Could you check a few things on this model? Use its own coordinates, in mm. Give positions to 0.01 mm unless a question says otherwise; leave off trailing zeros. Write each loop counter-clockwise with the first axis right and the second up, starting at its lowest first coordinate (ties: lowest second). Pieces come first, ordered by that corner, then holes. Notation, with made-up numbers: (58.5, 26.5) -> (90.5, 26.5) arc R12 cw to (90.5, 47.5) -> close; hole circle Ø5 at (-27.5, -22). An arc over 180 degrees is marked (long way). One line per question, with ' | ' between items.
from build123d import *

# Parameters (mm, degrees)
ESQUISSE1_W             = 370
ESQUISSE1_H             = 180
BOSS_EXTRU_1_DEPTH      = 6
ESQUISSE2_W             = 6
ESQUISSE2_H             = 30
ENL_V_MAT_EXTRU_1_DEPTH = 10
CONG_1_R                = 10


with BuildPart() as part:
    # Esquisse1 → Boss.-Extru.1 (new body)
    with BuildSketch(Plane.XY):
        with Locations((185, 90)):
            Rectangle(ESQUISSE1_W, ESQUISSE1_H)
    extrude(amount=BOSS_EXTRU_1_DEPTH)

    # Esquisse2 → Enlèv. mat.-Extru.1 (cut)
    with BuildSketch(Plane.XY.offset(6)):
        with Locations((8, 55)):
            Rectangle(ESQUISSE2_W, ESQUISSE2_H)
        with Locations((8, 125)):
            Rectangle(ESQUISSE2_W, ESQUISSE2_H)
        with Locations((362, 125)):
            Rectangle(ESQUISSE2_W, ESQUISSE2_H)
        with Locations((362, 55)):
            Rectangle(ESQUISSE2_W, ESQUISSE2_H)
    extrude(amount=-ENL_V_MAT_EXTRU_1_DEPTH, mode=Mode.SUBTRACT)

    # Congé1
    cong_1_edges = [part.edges().sort_by_distance(p)[0] for p in [
        (0, 180, 3),
        (370, 180, 3),
        (370, 0, 3),
        (0, 0, 3),
    ]]
    fillet(cong_1_edges, radius=CONG_1_R)


solid = part.part
Q1. Will these pins go through, and if not, where does the flat tip stop? pin 1 (1.8 mm diameter, centred on x = 363.5, z = 4, fed in from +Y); pin 2 (3 mm diameter, centred on x = 363, z = 1.5, fed in from -Y); pin 3 (1.8 mm diameter, centred on x = 7, z = 1.5, fed in from -Y).
Answer below:
pin 1: stops at y = 179.66 | pin 2: stops at y = 0.11 | pin 3: stops at y = 0.22
Q2. If I drill on line 1 along X through (y, z) = (124.5, 3.9), over which ranges is the centre line in solid material (lowest first)?
Answer below:
line 1: x = 0 to 5, 11 to 359, 365 to 370
Q3. Imagine slicing it at A-A on y = 117. Please give me the cut outline in (x, z), and give its area (3 significant figures).
Answer below:
outline: (0, 0) -> (5, 0) -> (5, 6) -> (0, 6) -> close; (11, 0) -> (359, 0) -> (359, 6) -> (11, 6) -> close; (365, 0) -> (370, 0) -> (370, 6) -> (365, 6) -> close | area: 2,150 mm^2
